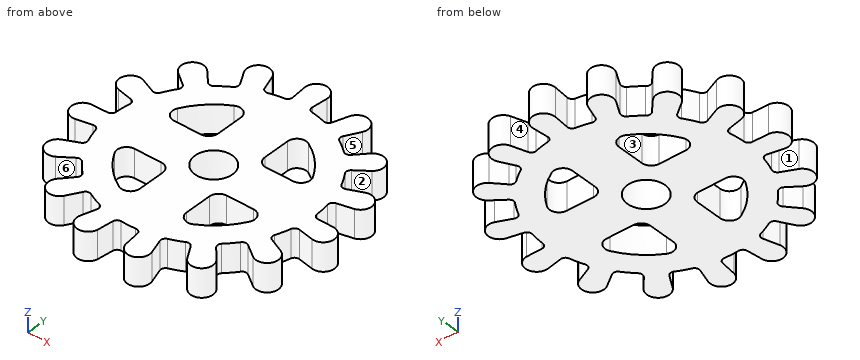
from build123d import *

# Parameters (mm, degrees)
F0_R     = 4
F1_DEPTH = 6


with BuildPart() as f1:
    # F0 (on Top) → F1 (new body)
    with BuildSketch(Plane.XY):
        with BuildLine():
            ThreePointArc((2.397418, 25.763696), (0, 28.275), (-2.397418, 25.763696))
            Line((-2.397418, 25.763696), (-2.087027, 22.428106))
            ThreePointArc((-2.087027, 22.428106), (-2.276181, 21.717887), (-2.899715, 21.32879))
            ThreePointArc((-2.899715, 21.32879), (-4.431874, 21.063811), (-5.940908, 20.688916))
            ThreePointArc((-5.940908, 20.688916), (-6.714959, 20.745067), (-7.215738, 21.337965))
            Line((-7.215738, 21.337965), (-8.288889, 24.511425))
            ThreePointArc((-8.288889, 24.511425), (-11.500479, 25.830498), (-12.669189, 22.56119))
            Line((-12.669189, 22.56119), (-11.028927, 19.640224))
            ThreePointArc((-11.028927, 19.640224), (-10.912855, 18.914471), (-11.324222, 18.305399))
            ThreePointArc((-11.324222, 18.305399), (-12.616142, 17.440143), (-13.842229, 16.48388))
            ThreePointArc((-13.842229, 16.48388), (-14.572199, 16.220342), (-15.270837, 16.558296))
            Line((-15.270837, 16.558296), (-17.541972, 19.020906))
            ThreePointArc((-17.541972, 19.020906), (-21.01242, 18.919668), (-20.750343, 15.457649))
            Line((-20.750343, 15.457649), (-18.063825, 13.456369))
            ThreePointArc((-18.063825, 13.456369), (-17.662597, 12.840571), (-17.790668, 12.116838))
            ThreePointArc((-17.790668, 12.116838), (-18.618965, 10.800916), (-19.350104, 9.428632))
            ThreePointArc((-19.350104, 9.428632), (-19.909774, 8.890972), (-20.68547, 8.915547))
            Line((-20.68547, 8.915547), (-23.761888, 10.241499))
            ThreePointArc((-23.761888, 10.241499), (-26.891123, 8.737456), (-25.243573, 5.68134))
            Line((-25.243573, 5.68134), (-21.975323, 4.945785))
            ThreePointArc((-21.975323, 4.945785), (-21.358316, 4.546419), (-21.180946, 3.833166))
            ThreePointArc((-21.180946, 3.833166), (-21.402399, 2.294112), (-21.51217, 0.743088))
            ThreePointArc((-21.51217, 0.743088), (-21.804767, 0.024273), (-22.523396, -0.268781))
            Line((-22.523396, -0.268781), (-25.873158, -0.308755))
            ThreePointArc((-25.873158, -0.308755), (-28.120107, -2.955542), (-25.371961, -5.077324))
            Line((-25.371961, -5.077324), (-22.087089, -4.41997))
            ThreePointArc((-22.087089, -4.41997), (-21.360988, -4.533849), (-20.908846, -5.113295))
            ThreePointArc((-20.908846, -5.113295), (-20.485164, -6.609364), (-19.954586, -8.070943))
            ThreePointArc((-19.954586, -8.070943), (-19.929519, -8.846624), (-20.466823, -9.406634))
            Line((-20.466823, -9.406634), (-23.510724, -10.805623))
            ThreePointArc((-23.510724, -10.805623), (-24.486868, -14.1375), (-21.113306, -14.958072))
            Line((-21.113306, -14.958072), (-18.379796, -13.021472))
            ThreePointArc((-18.379796, -13.021472), (-17.670151, -12.830174), (-17.021417, -13.175622))
            ThreePointArc((-17.021417, -13.175622), (-16.025858, -14.370021), (-14.946673, -15.489435))
            ThreePointArc((-14.946673, -15.489435), (-14.608275, -16.187858), (-14.871351, -16.917995))
            Line((-14.871351, -16.917995), (-17.083072, -19.434101))
            ThreePointArc((-17.083072, -19.434101), (-16.619628, -22.874956), (-13.203969, -22.252434))
            Line((-13.203969, -22.252434), (-11.494469, -19.371443))
            ThreePointArc((-11.494469, -19.371443), (-10.923984, -18.908045), (-10.19083, -18.959763))
            ThreePointArc((-10.19083, -18.959763), (-8.795535, -19.645971), (-7.354344, -20.229662))
            ThreePointArc((-7.354344, -20.229662), (-6.761128, -20.730065), (-6.704486, -21.504081))
            Line((-6.704486, -21.504081), (-7.701602, -24.702246))
            ThreePointArc((-7.701602, -24.702246), (-5.878703, -27.657123), (-3.011545, -25.699148))
            Line((-3.011545, -25.699148), (-2.621645, -22.371916))
            ThreePointArc((-2.621645, -22.371916), (-2.288962, -21.716543), (-1.598156, -21.465589))
            ThreePointArc((-1.598156, -21.465589), (-0.044385, -21.524954), (1.509617, -21.471998))
            ThreePointArc((1.509617, -21.471998), (2.255079, -21.687856), (2.621645, -22.371916))
            Line((2.621645, -22.371916), (3.011545, -25.699148))
            ThreePointArc((3.011545, -25.699148), (5.878703, -27.657123), (7.701602, -24.702246))
            Line((7.701602, -24.702246), (6.704486, -21.504081))
            ThreePointArc((6.704486, -21.504081), (6.741843, -20.770054), (7.270854, -20.25982))
            ThreePointArc((7.270854, -20.25982), (8.71444, -19.682077), (10.112552, -19.001629))
            ThreePointArc((10.112552, -19.001629), (10.881363, -18.895619), (11.494469, -19.371443))
            Line((11.494469, -19.371443), (13.203969, -22.252434))
            ThreePointArc((13.203969, -22.252434), (16.619628, -22.874956), (17.083072, -19.434101))
            Line((17.083072, -19.434101), (14.871351, -16.917995))
            ThreePointArc((14.871351, -16.917995), (14.606923, -16.232234), (14.882667, -15.550944))
            ThreePointArc((14.882667, -15.550944), (15.966459, -14.43599), (16.966935, -13.245707))
            ThreePointArc((16.966935, -13.245707), (17.62616, -12.836158), (18.379796, -13.021472))
            Line((18.379796, -13.021472), (21.113306, -14.958072))
            ThreePointArc((21.113306, -14.958072), (24.486868, -14.1375), (23.510724, -10.805623))
            Line((23.510724, -10.805623), (20.466823, -9.406634))
            ThreePointArc((20.466823, -9.406634), (19.946332, -8.887713), (19.921131, -8.153168))
            ThreePointArc((19.921131, -8.153168), (20.457732, -6.693789), (20.887581, -5.199481))
            ThreePointArc((20.887581, -5.199481), (21.323234, -4.557208), (22.087089, -4.41997))
            Line((22.087089, -4.41997), (25.371961, -5.077324))
            ThreePointArc((25.371961, -5.077324), (28.120107, -2.955542), (25.873158, -0.308755))
            Line((25.873158, -0.308755), (22.523396, -0.268781))
            ThreePointArc((22.523396, -0.268781), (21.83684, -0.006426), (21.515051, 0.654364))
            ThreePointArc((21.515051, 0.654364), (21.411678, 2.205828), (21.196574, 3.745782))
            ThreePointArc((21.196574, 3.745782), (21.333327, 4.509724), (21.975323, 4.945785))
            Line((21.975323, 4.945785), (25.243573, 5.68134))
            ThreePointArc((25.243573, 5.68134), (26.891123, 8.737456), (23.761888, 10.241499))
            Line((23.761888, 10.241499), (20.68547, 8.915547))
            ThreePointArc((20.68547, 8.915547), (19.951559, 8.875973), (19.388824, 9.348751))
            ThreePointArc((19.388824, 9.348751), (18.66335, 10.724038), (17.840487, 12.043366))
            ThreePointArc((17.840487, 12.043366), (17.654695, 12.796884), (18.063825, 13.456369))
            Line((18.063825, 13.456369), (20.750343, 15.457649))
            ThreePointArc((20.750343, 15.457649), (21.01242, 18.919668), (17.541972, 19.020906))
            Line((17.541972, 19.020906), (15.270837, 16.558296))
            ThreePointArc((15.270837, 16.558296), (14.616473, 16.223635), (13.910092, 16.426654))
            ThreePointArc((13.910092, 16.426654), (12.687959, 17.387965), (11.399618, 18.258542))
            ThreePointArc((11.399618, 18.258542), (10.923405, 18.871346), (11.028927, 19.640224))
            Line((11.028927, 19.640224), (12.669189, 22.56119))
            ThreePointArc((12.669189, 22.56119), (11.500479, 25.830498), (8.288889, 24.511425))
            Line((8.288889, 24.511425), (7.215738, 21.337965))
            ThreePointArc((7.215738, 21.337965), (6.754066, 20.766083), (6.026179, 20.664239))
            ThreePointArc((6.026179, 20.664239), (4.518705, 21.045354), (2.987651, 21.31665))
            ThreePointArc((2.987651, 21.31665), (2.303359, 21.682781), (2.087027, 22.428106))
            Line((2.087027, 22.428106), (2.397418, 25.763696))
        make_face()
        with BuildLine():
            ThreePointArc((-14.479386, -7.963855), (-14.44855, -5.982088), (-12.726964, -5))
            Line((-12.726964, -5), (-7, -5))
            ThreePointArc((-7, -5), (-5.585786, -5.585786), (-5, -7))
            Line((-5, -7), (-5, -12.726964))
            ThreePointArc((-5, -12.726964), (-5.982088, -14.44855), (-7.963855, -14.479386))
            ThreePointArc((-7.963855, -14.479386), (-11.68494, -11.68494), (-14.479386, -7.963855))
        make_face(mode=Mode.SUBTRACT)
        with BuildLine():
            ThreePointArc((7.963855, -14.479386), (5.982088, -14.44855), (5, -12.726964))
            Line((5, -12.726964), (5, -7))
            ThreePointArc((5, -7), (5.585786, -5.585786), (7, -5))
            Line((7, -5), (12.726964, -5))
            ThreePointArc((12.726964, -5), (14.44855, -5.982088), (14.479386, -7.963855))
            ThreePointArc((14.479386, -7.963855), (11.68494, -11.68494), (7.963855, -14.479386))
        make_face(mode=Mode.SUBTRACT)
        Circle(F0_R, mode=Mode.SUBTRACT)
        with BuildLine():
            ThreePointArc((-7.963855, 14.479386), (-5.982088, 14.44855), (-5, 12.726964))
            Line((-5, 12.726964), (-5, 7))
            ThreePointArc((-5, 7), (-5.585786, 5.585786), (-7, 5))
            Line((-7, 5), (-12.726964, 5))
            ThreePointArc((-12.726964, 5), (-14.44855, 5.982088), (-14.479386, 7.963855))
            ThreePointArc((-14.479386, 7.963855), (-11.68494, 11.68494), (-7.963855, 14.479386))
        make_face(mode=Mode.SUBTRACT)
        with BuildLine():
            ThreePointArc((14.479386, 7.963855), (14.44855, 5.982088), (12.726964, 5))
            Line((12.726964, 5), (7, 5))
            ThreePointArc((7, 5), (5.585786, 5.585786), (5, 7))
            Line((5, 7), (5, 12.726964))
            ThreePointArc((5, 12.726964), (5.982088, 14.44855), (7.963855, 14.479386))
            ThreePointArc((7.963855, 14.479386), (11.68494, 11.68494), (14.479386, 7.963855))
        make_face(mode=Mode.SUBTRACT)
    extrude(amount=F1_DEPTH)


solid = f1.part
Model file for the job. Use its own axes, mm. Face numbers are marked on the shaded views. A direction names the side the tool comes from. Round coordinates to 2 decimals unless told otherwise and drop trailing zeros. Order: outer loops, then holes, each group sorted by start corner. A loop starts at its lowest first (then second) coordinate and runs counter-clockwise, first axis right, second up. Notation, with made-up numbers: M 85.25,-15 L 122.25,-15 A19 ccw 122.25,4 Z; hole C -23.75,-32 d7. An arc over 180 degrees is marked long. Write each question's results on one line, items separated by ' | '. Start each with the question number.
(1) Saw through at A-A, the plane x = 0. Give the cut face in (y, z) (3 decimals).
(2) Drop flat-ended pins along their axis: pin 1 (1.5 mm diameter, centred on y = 22, z = 5, fed in from -X); pin 2 (8 mm diameter, centred on x = -4, y = 7.5, fed in from -Z); pin 3 (1.7 mm diameter, centred on y = 11, z = 4, fed in from +X); pin 4 (3 mm diameter, centred on x = 9, z = 4, fed in from +Y). Give the stop position or say it passes through.
(3) Which spindle directions (+Z, -Z, +X, -X, +Y, -Y) get a long thin tool onto all of the face, cutting with end or side? Do the marked faces 1, 2 and 3. Say none if no direction does.
(4) Saw through at C-C, the plane z = 2.85. State how many separate pieces and enclosed holes the cut face has, then the cut area to 3 significant figures.
(5) Two-plate mould, pull along Y, no slides. Class the marked faces 4, 5 and 6: pulls with the +Y half, pulls with the -Y half, needs draft (parallel to the pull), parting line crosses it, or undercut.
(6) Saw through at B-B, the plane y = 2. Give the cut face in (x, z).
(7) Probe probe 1 along X at (y, z) = (19.5, 2.05); probe 2 along Y at (x, z) = (-5.5, 2.8); probe 3 along X at (y, z) = (14, 2.25). List the from-to ranges inside material, lowest first. Write a range as from..to.
Established:
1) outline: M -21.525,0 L -4,0 L -4,6 L -21.525,6 Z; M 4,0 L 28.275,0 L 28.275,6 L 4,6 Z
2) pin 1: stops at x = -12.75 | pin 2: stops at z = 0 | pin 3: stops at x = 25.67 | pin 4: stops at y = 26.04
3) face 1: +Z, -Z, -X | face 2: +Z, -Z, +X | face 3: +Z, -Z
4) separate pieces: 1 | enclosed holes: 5 | area: 1,550 mm^2
5) face 4: pulls with the +Y half | face 5: undercut | face 6: pulls with the -Y half
6) outline: M -21.43,0 L -3.46,0 L -3.46,6 L -21.43,6 Z; M 3.46,0 L 21.43,0 L 21.43,6 L 3.46,6 Z
7) probe 1: x = -20.22..-18.24, -10.96..10.96, 18.24..20.22 | probe 2: y = -27.71..-14.05, -5.68..5.68, 14.05..20.81 | probe 3: x = -18.79..-8.78, -5.46..5.46, 8.78..18.79
